Model file for the job. Use its own axes, mm. Face numbers are marked on the shaded views. A direction names the side the tool comes from. Coordinates: 2 decimals unless noted, no trailing zeros. Loops run counter-clockwise (first coordinate to the right, second up) from the corner with the lowest first, then second, coordinate; pieces in that order, holes last.
from build123d import *

# Parameters (mm, degrees)
BOSS_EXTRUDE1_START      = -4
SKETCH8_R                = 4
BOSS_EXTRUDE1_DEPTH      = 4
BOSS_EXTRUDE2_DEPTH      = 7
BOSS_EXTRUDE2_DEPTH_BACK = 100
SKETCH7_2_R              = 6


with BuildPart() as part:
    # Sketch1 → Revolve1 (revolve)
    with BuildSketch(Plane.XY, mode=Mode.PRIVATE) as revolve1_sk:
        Polygon((-25, 22), (-25, 17), (-13, 17), (-13, 15), (13, 15), (13, 17), (25, 17), (25, 22), align=None)
    revolve(revolve1_sk.sketch.rotate(Axis((-45.766103365, 0, 0), (1, 0, 0)), 90), axis=Axis((-45.766103365, 0, 0), (1, 0, 0)))

    # Sketch8 → Boss-Extrude1 (add)
    with BuildSketch(Plane(origin=(25, 0, 0), x_dir=(0, 0, -1), z_dir=(1, 0, 0)).offset(BOSS_EXTRUDE1_START)):
        with BuildLine():
            Line((-22, 0), (-57, 0))
            Line((-57, 0), (-57, 15.102123796))
            Line((-57, 15.102123796), (-76.188059939, 15.102123796))
            Line((-76.188059939, 15.102123796), (-76.188059939, -14.897876204))
            Line((-76.188059939, -14.897876204), (-16.188059939, -14.897876204))
            ThreePointArc((-16.188059939, -14.897876204), (-20.49557658, -7.99570764), (-22, 0))
        make_face()
        with Locations((-66.724926484, 6.517856695)):
            Circle(SKETCH8_R, mode=Mode.SUBTRACT)
    extrude(amount=BOSS_EXTRUDE1_DEPTH)

    # Sketch7_2 → Boss-Extrude2 (add, two sides: drawn at the far end of the back side and taken through both)
    with BuildSketch(Plane(origin=(-2.661140852, -21.673252989, 0), x_dir=(0, 0, -1), z_dir=(0.1218693434051474, 0.9925461516413221, 0)).offset(-BOSS_EXTRUDE2_DEPTH_BACK)):
        with Locations(Location((0, -2.681125555, 0), (0, 0, 90))):
            Circle(SKETCH7_2_R)
    extrude(amount=BOSS_EXTRUDE2_DEPTH + BOSS_EXTRUDE2_DEPTH_BACK)


solid = part.part
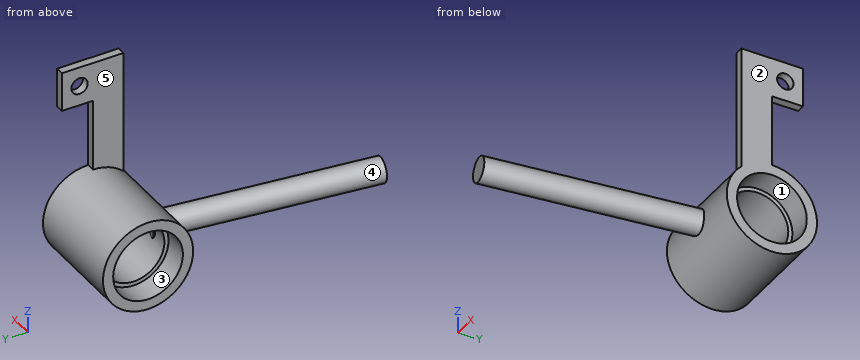
Q1. Slice it at D-D (z = 69). List the corners of the cut face in (x, y), and give its area (3 significant figures).
Answers:
outline: (21, -14.9) - (25, -14.9) - (25, 3.23) - (21, 3.23) - close; (21, 9.81) - (25, 9.81) - (25, 15.1) - (21, 15.1) - close
area: 93.7 mm2
Q2. Which spindle directions (+Z, -Z, +X, -X, +Y, -Y) get a long thin tool onto all of the face, cutting with end or side? Do the marked faces 1, 2 and 3. Say none if no direction does.
Answers:
face 1: +X
face 2: +Z, -Z, +X, +Y, -Y
face 3: -X
Q3. Slice it at B-B (x = 10). List the corners of the cut face in (y, z), and give its area (3 significant figures).
Answers:
outline: circle Ø44 at (0, 0); hole circle Ø30 at (0, 0)
area: 814 mm2
Q4. Flat gauge pins, fed straight in: P1, Ø17, axis at y = -5, z = -5, coming from the +X side; P2, Ø12, axis at x = 13.5, y = -53, coming from the +Z side; P3, Ø2, axis at x = 24, y = 10.5, coming from the -Z side; P4, Ø4.5, axis at x = 24, z = 69, coming from the +Y side. Where does each tip first touch, or does it go through?
Answers:
P1: stops at x = 13
P2: passes through
P3: stops at z = -19.84
P4: stops at y = 15.1
Q5. Slice it at C-C (z = 49.5). List the corners of the cut face in (x, y).
Answers:
outline: (21, -14.9) - (25, -14.9) - (25, 0) - (21, 0) - close
Q6. Drill centre lines: line 1 (Y direction, x = 22, z = 0); line 2 (Y direction, x = -17, z = -13); line 3 (Z direction, x = 15, y = 14.5). Where is each one in solid material? Low to high.
Answers:
line 1: y = -22 to -17, 17 to 22
line 2: y = -17.75 to -10.95, 10.95 to 17.75
line 3: z = -16.55 to -8.87, 8.87 to 16.55
Q7. Slice it at A-A (z = -13). List the corners of the cut face in (x, y), and give its area (3 significant figures).
Answers:
outline: (-25, -17.75) - (25, -17.75) - (25, -10.95) - (13, -10.95) - (13, -7.48) - (-13, -7.48) - (-13, -10.95) - (-25, -10.95) - close; (-25, 10.95) - (-13, 10.95) - (-13, 7.48) - (13, 7.48) - (13, 10.95) - (25, 10.95) - (25, 17.75) - (-25, 17.75) - close
area: 860 mm2
Q8. Mould opens along Y. For the marked faces 4 and 5 say: +Y half, -Y half, draft (parallel to the pull), parting line (faces both ways), or undercut.
Answers:
face 4: undercut
face 5: draft
